from build123d import *

# Parameters (mm, degrees)
SKETCH1_W           = 240
SKETCH1_H           = 30
BOSS_EXTRUDE1_DEPTH = 4
SKETCH2_R           = 4.25
CUT_EXTRUDE1_DEPTH  = 242.900806117
SKETCH3_R           = 8
CUT_EXTRUDE2_DEPTH  = 242.900806117


with BuildPart() as part:
    # Sketch1 → Boss-Extrude1 (new body)
    with BuildSketch(Plane.XY):
        with Locations((120, 15)):
            Rectangle(SKETCH1_W, SKETCH1_H)
    extrude(amount=BOSS_EXTRUDE1_DEPTH)

    # Sketch2 → Cut-Extrude1 (cut, through all)
    with BuildSketch(Plane.XY.offset(4)):
        with Locations((225, 15)):
            Circle(SKETCH2_R)
        with Locations((15, 15)):
            Circle(SKETCH2_R)
    extrude(amount=-CUT_EXTRUDE1_DEPTH, mode=Mode.SUBTRACT)

    # Sketch3 → Cut-Extrude2 (cut, through all)
    with BuildSketch(Plane(origin=(0, 0, 0), x_dir=(-1, 0, 0), z_dir=(0, 0, -1))):
        with Locations((-90, 15)):
            Circle(SKETCH3_R)
    extrude(amount=-CUT_EXTRUDE2_DEPTH, mode=Mode.SUBTRACT)


solid = part.part
Read the model definition and answer for the solid it produces. Units are mm, in the model's axes. Round coordinates to 2 decimals unless told otherwise and drop trailing zeros. Write each loop counter-clockwise with the first axis right and the second up, starting at its lowest first coordinate (ties: lowest second). Pieces come first, ordered by that corner, then holes. Notation, with made-up numbers: M 54.5,27 L 96.5,27 A9 cw 96.5,33 Z; hole C 46.25,83 d6. An arc over 180 degrees is marked long. Use a Markdown table: item, result.
1) Straight lines are drawn through the part: line 1 along X through (y, z) = (14.75, 1); line 2 along Y through (x, z) = (225, 1.5); line 3 along X through (y, z) = (12.5, 3.55). For each, find the intervals that lie inside material, in ascending order. Write a range as [from, to].
Answers follow:
| item | result |
|---|---|
| line 1 | x = [0, 10.76], [19.24, 82], [98, 220.76], [229.24, 240] |
| line 2 | y = [0, 10.75], [19.25, 30] |
| line 3 | x = [0, 11.56], [18.44, 82.4], [97.6, 221.56], [228.44, 240] |
2) The part is cut by section D-D (x = 15). Write down the section's boundary in (y, z), plus the area to 3 significant figures.
Answers follow:
| item | result |
|---|---|
| outline | M 0,0 L 10.75,0 L 10.75,4 L 0,4 Z; M 19.25,0 L 30,0 L 30,4 L 19.25,4 Z |
| area | 86.0 mm2 |
3) The part is cut by section C-C (z = 1.4). Write down the section's boundary in (x, y), plus the area to 3 significant figures.
Answers follow:
| item | result |
|---|---|
| outline | M 0,0 L 240,0 L 240,30 L 0,30 Z; hole C 15,15 d8.5; hole C 90,15 d16; hole C 225,15 d8.5 |
| area | 6,890 mm2 |
4) The part is cut by section A-A (x = 90). Write down the section's boundary in (y, z).
Answers follow:
| item | result |
|---|---|
| outline | M 0,0 L 7,0 L 7,4 L 0,4 Z; M 23,0 L 30,0 L 30,4 L 23,4 Z |
5) The part is cut by section B-B (y = 15). Write down the section's boundary in (x, z).
Answers follow:
| item | result |
|---|---|
| outline | M 0,0 L 10.75,0 L 10.75,4 L 0,4 Z; M 19.25,0 L 82,0 L 82,4 L 19.25,4 Z; M 98,0 L 220.75,0 L 220.75,4 L 98,4 Z; M 229.25,0 L 240,0 L 240,4 L 229.25,4 Z |
6) For a pull along X with two mould halves and no side action, classify faces 1 (the flat face through (118, 30, 2)), 2 (the flat face through (0, 15, 2)), 3 (the cylindrical face through (221.63, 12.41, 2.03)) as pulls with the +X half, pulls with the -X half, needs draft (parallel to the pull), parting line crosses it, or undercut.
Answers follow:
| item | result |
|---|---|
| face 1 | needs draft |
| face 2 | pulls with the -X half |
| face 3 | undercut |
